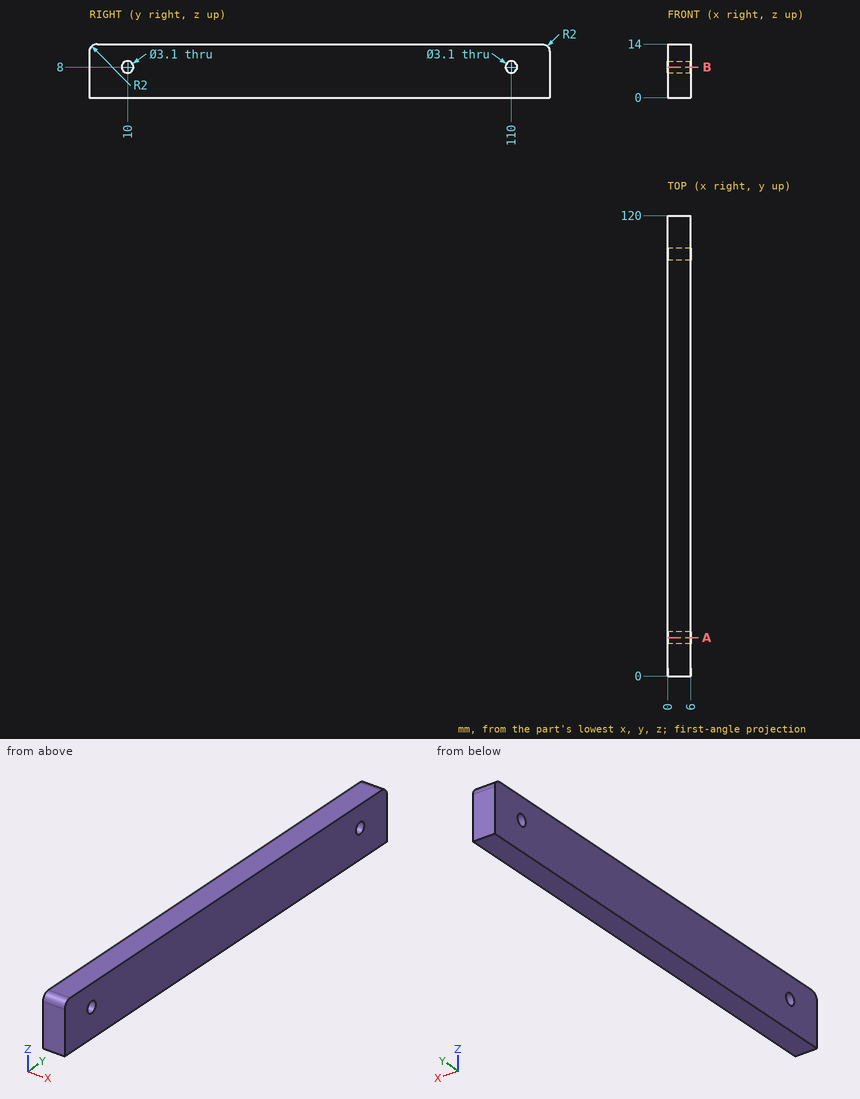
Source: three-view drawing plus pictorial views. Frame: mm from the lowest corner of the part. Round coordinates to 2 decimals unless told otherwise and drop trailing zeros. Write each loop counter-clockwise with the first axis right and the second up, starting at its lowest first coordinate (ties: lowest second). Pieces come first, ordered by that corner, then holes. Notation, with made-up numbers: M 43.25,2.5 L 61.25,2.5 A7 ccw 61.25,6.5 Z; hole C 57.25,49.25 d2. An arc over 180 degrees is marked long. One line per item, written item: value. Start each with the question number.
Item 1: Section query A-A (y = 10). Return the cut outline in (x, z).
Item 2: Section query B-B (z = 8). Return the cut outline in (x, y).
Item 3: Pin query (flat end, axial travel): pin 1 (3 mm diameter, centred on y = 10, z = 8, fed in from +X). Return the tip coordinate at first contact, or that it passes through.
Item 4: Ray query, L1, parallel to Y at x = 3.3, z = 8; L2, parallel to Z at x = 3.75, y = 110; L3, parallel to Z at x = 2.55, y = 109. Return the intervals inside material, ascending. Write a range as from..to.
Result set:
1. outline: M 0,0 L 6,0 L 6,6.45 L 0,6.45 Z; M 0,9.55 L 6,9.55 L 6,14 L 0,14 Z
2. outline: M 0,0 L 6,0 L 6,8.45 L 0,8.45 Z; M 0,11.55 L 6,11.55 L 6,108.45 L 0,108.45 Z; M 0,111.55 L 6,111.55 L 6,120 L 0,120 Z
3. pin 1: passes through
4. L1: y = 0..8.45, 11.55..108.45, 111.55..120
4. L2: z = 0..6.45, 9.55..14
4. L3: z = 0..6.82, 9.18..14
